from build123d import *

# Parameters (mm, degrees)
SKETCH2_W               = 8
SKETCH2_H               = 13
SKETCH2_H_2             = 10
CUT_EXTRUDE1_DEPTH      = 24.938835821
CUT_EXTRUDE2_DEPTH      = 24.938835821
CUT_EXTRUDE2_DEPTH_BACK = 24.938835821
SKETCH3_R               = 1.5
CUT_EXTRUDE3_DEPTH      = 10
CUT_EXTRUDE3_DEPTH_BACK = 10


with BuildPart() as part:
    # Sketch1 → Revolve1 (revolve)
    with BuildSketch(Plane(origin=(0, 0, 0), x_dir=(0, 0, -1), z_dir=(1, 0, 0))):
        with BuildLine():
            Line((0, 20), (0, -20))
            Line((0, -20), (8, -20))
            add(Edge.make_bspline(
                [(8, 20), (10.604722665, 5.227883705), (8, -20)],
                knots=[0, 0, 0, 1, 1, 1], degree=2))
            Line((8, 20), (0, 20))
        make_face()
    revolve(axis=Axis((0, 20, 0), (0, -1, 0)))

    # Sketch2 → Cut-Extrude1 (cut, through all)
    with BuildSketch(Plane(origin=(0, 0, 0), x_dir=(0, 0, -1), z_dir=(1, 0, 0))):
        with Locations((0, 13.5)):
            Rectangle(SKETCH2_W, SKETCH2_H)
        with Locations((0, -15)):
            Rectangle(SKETCH2_W, SKETCH2_H_2)
    extrude(amount=-CUT_EXTRUDE1_DEPTH, mode=Mode.SUBTRACT)

    # Sketch3 → Cut-Extrude2 (cut, two sides: drawn at the far end of the back side and taken through both)
    with BuildSketch(Plane.XY.offset(-CUT_EXTRUDE2_DEPTH_BACK)):
        with Locations((-3.464101615, 15)):
            Circle(SKETCH3_R)
        with Locations((-3.464101615, -15)):
            Circle(SKETCH3_R)
    extrude(amount=CUT_EXTRUDE2_DEPTH + CUT_EXTRUDE2_DEPTH_BACK, mode=Mode.SUBTRACT)

    # Sketch4 → Cut-Extrude3 (cut, two sides: drawn at the far end of the back side and taken through both)
    with BuildSketch(Plane.XY.offset(-CUT_EXTRUDE3_DEPTH_BACK)):
        with BuildLine():
            Line((-2, 20), (9.10519633, 10))
            add(Edge.make_bspline(
                [(9.10519633, 10), (8.795626613, 15.487777253), (8, 20)],
                knots=[0.694544596, 0.694544596, 0.694544596, 1, 1, 1], degree=2))
            Line((8, 20), (-2, 20))
        make_face()
    extrude(amount=CUT_EXTRUDE3_DEPTH + CUT_EXTRUDE3_DEPTH_BACK, mode=Mode.SUBTRACT)


solid = part.part
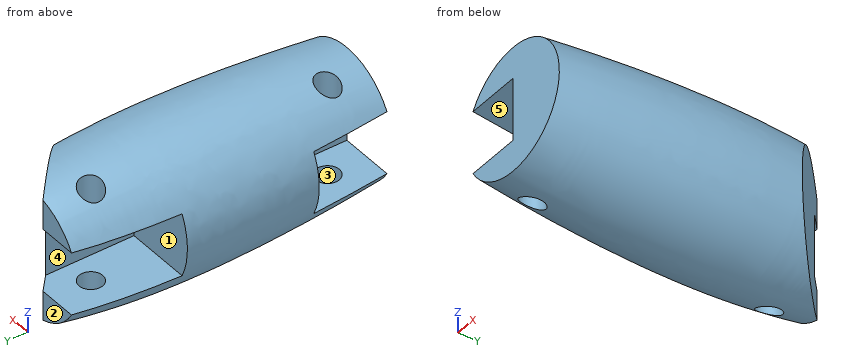
Work out the finished part from the listing and answer in its coordinate system (mm). Face numbers are marked on the shaded views. A direction names the side the tool comes from. Give positions to 0.01 mm unless a question says otherwise; leave off trailing zeros. Use a Markdown table: item, result. Add a question column.
1. Find the intervals of material crossed by probe 1 along Y at (x, z) = (-2.5, -5.25); probe 2 along X at (y, z) = (15, 6.2); probe 3 along Y at (x, z) = (-7.5, 3), in increasing order.
2. Flat-ended cylindrical pins translate along their axes: pin 1 Ø3 at (x, y) = (0.5, 5) entering from -Z; pin 2 Ø2.5 at (x, y) = (-3, 14) entering from +Z; pin 3 Ø10 at (y, z) = (-3.5, 5.5) entering from +X; pin 4 Ø2.5 at (x, y) = (-3.46, 15) entering from +Z. Find the tip coordinate at first contact, or state that the pin passes through.
3. For the marked faces 3, 4 and 5, determine the directions among +Z, -Z, +X, -X, +Y, -Y from which every point of the face is accessible in a straight line to the end or side of a thin tool.
4. Section A-A on y = 14 is taken. State how many separate pieces and enclosed holes the cut face has, and give its area (3 significant figures).
5. Determine the mould class of the marked faces 1 and 2 for opening direction Z: released by +Z, released by -Z, zero draft, split by the parting line, or undercut.
Results below:
| question | item | result |
|---|---|---|
| 1 | probe 1 | y = -20 to -16.15, -13.85 to 13.85, 16.15 to 20 |
| 1 | probe 2 | x = -6.1 to -4.96, -1.96 to 3.55 |
| 1 | probe 3 | y = -10 to 7 |
| 2 | pin 1 | stops at z = -9.3 |
| 2 | pin 2 | stops at z = 8.65 |
| 2 | pin 3 | stops at x = 9.21 |
| 2 | pin 4 | passes through |
| 3 | face 3 | +Z, -Z |
| 3 | face 4 | -X, +Y |
| 3 | face 5 | -X, -Y |
| 4 | separate pieces | 3 |
| 4 | enclosed holes | 0 |
| 4 | area | 114 mm^2 |
| 5 | face 1 | undercut |
| 5 | face 2 | zero draft |
